Read the model definition and answer for the solid it produces. Units are mm, in the model's axes. Round coordinates to 2 decimals unless told otherwise and drop trailing zeros. Order: outer loops, then holes, each group sorted by start corner. A loop starts at its lowest first (then second) coordinate and runs counter-clockwise, first axis right, second up. Notation, with made-up numbers: (-31, -36.5) -> (-1, -36.5) arc R33 cw to (-1, -2.5) -> close; hole circle Ø10 at (-40, 35.5). An arc over 180 degrees is marked (long way). Answer as a JSON object with one key per item and string values. Group by question number.
Item 1: Given P1, Ø2, axis at x = 106.5, z = 5, coming from the +Y side; P2, Ø1, axis at y = 34, z = 4, coming from the -X side, each flat-ended and moving along its own axis, determine where each tip first touches the part or whether it passes through.
Item 2: Section A-A, the plane y = 2.5 is taken. Write down the section's boundary in (x, z).
Item 3: Section B-B, the plane x = 21.5 is taken. Write down the section's boundary in (y, z), plus the area to 3 significant figures.
Item 4: Consider probe 1 along X at (y, z) = (0.5, 5.75); probe 2 along Y at (x, z) = (105.5, 1.5); probe 3 along Y at (x, z) = (21, 4.5). Determine where each line is inside the solid, lowest interval first. Write a range as from..to.
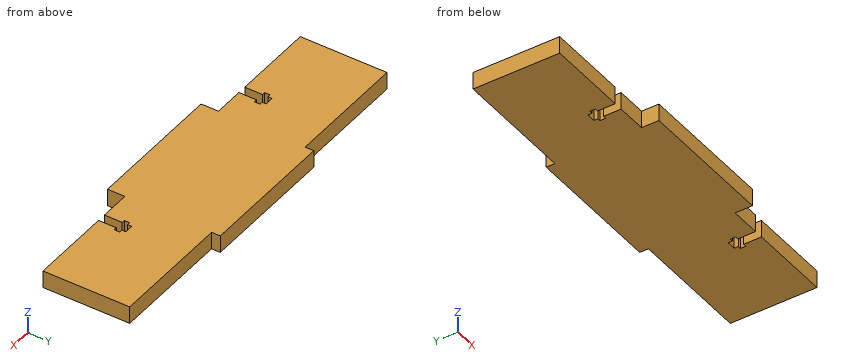
from build123d import *

# Parameters (mm, degrees)
BOSS_EXTRUDE1_DEPTH = 6.35
CUT_EXTRUDE1_DEPTH  = 7.35


with BuildPart() as part:
    # Sketch1 → Boss-Extrude1 (new body)
    with BuildSketch(Plane.XY):
        Polygon((0, 0), (44.45, 0), (44.45, -6.35), (95.25, -6.35), (95.25, 0), (139.7, 0), (139.7, 31.75), (95.25, 31.75), (95.25, 34.925), (44.45, 34.925), (44.45, 31.75), (0, 31.75), align=None)
    extrude(amount=BOSS_EXTRUDE1_DEPTH)

    # Sketch2 → Cut-Extrude1 (cut, through all)
    with BuildSketch(Plane.XY.offset(6.35)):
        Polygon((30.15, 0), (33.35, 0), (33.35, 6.5), (34.5, 6.5), (34.5, 8.5), (33.35, 8.5), (33.35, 10), (30.15, 10), (30.15, 8.5), (29, 8.5), (29, 6.5), (30.15, 6.5), align=None)
        Polygon((109.55, 8.5), (109.55, 10), (106.35, 10), (106.35, 8.5), (105.2, 8.5), (105.2, 6.5), (106.35, 6.5), (106.35, 0), (109.55, 0), (109.55, 6.5), (110.7, 6.5), (110.7, 8.5), align=None)
    extrude(amount=-CUT_EXTRUDE1_DEPTH, mode=Mode.SUBTRACT)


solid = part.part
Values found:
{
 "1": {"P1": "y = 31.75", "P2": "x = 44.45"},
 "2": {"outline": "(0, 0) -> (30.15, 0) -> (30.15, 6.35) -> (0, 6.35) -> close; (33.35, 0) -> (106.35, 0) -> (106.35, 6.35) -> (33.35, 6.35) -> close; (109.55, 0) -> (139.7, 0) -> (139.7, 6.35) -> (109.55, 6.35) -> close"},
 "3": {"outline": "(0, 0) -> (31.75, 0) -> (31.75, 6.35) -> (0, 6.35) -> close", "area": "202 mm2"},
 "4": {"probe 1": "0..30.15, 33.35..106.35, 109.55..139.7", "probe 2": "0..6.5, 8.5..31.75", "probe 3": "0..31.75"}
}
